Here's how the part is built. I have some questions about the finished solid (model axes, mm). Face numbers are marked on the shaded views. A direction names the side the tool comes from. Round coordinates to 2 decimals unless told otherwise and drop trailing zeros. Write each loop counter-clockwise with the first axis right and the second up, starting at its lowest first coordinate (ties: lowest second). Pieces come first, ordered by that corner, then holes. Notation, with made-up numbers: M 38.5,56.5 L 56.5,56.5 A15 ccw 56.5,83.5 Z; hole C -5.5,58.25 d11. An arc over 180 degrees is marked long. Use a Markdown table: item, result. Add a question column.
```python
from build123d import *

# Parameters (mm, degrees)
F1_DEPTH = 10
F0_R     = 38.1
F0_R_2   = 6.35
F0_R_3   = 5.8823611715
F2_DEPTH = 3
F0_R_4   = 4
F3_DEPTH = 6.35


with BuildPart() as f1:
    # F0 (on Top) → F1 (new body)
    with BuildSketch(Plane.XY):
        with BuildLine():
            Line((25.7629516235, 0), (28.75, 0))
            ThreePointArc((28.75, 0), (28.7346354423, 0.9398010419), (28.6885581914, 1.878597588))
            ThreePointArc((28.6885581914, 1.878597588), (27.1771412956, 2.3608673988), (25.7015098149, 1.7782209055))
            ThreePointArc((25.7015098149, 1.7782209055), (25.7475865895, 0.889641035), (25.7629516235, 0))
        make_face()
        with BuildLine():
            ThreePointArc((28.6885581914, 1.878597588), (28.7346354423, 0.9398010419), (28.75, 0))
            ThreePointArc((28.75, 0), (28.7346354423, -0.9398010419), (28.6885581914, -1.878597588))
            ThreePointArc((28.6885581914, -1.878597588), (29.3734139116, -1.0481230469), (29.6186758117, 0))
            ThreePointArc((29.6186758117, 0), (29.3734139116, 1.0481230469), (28.6885581914, 1.878597588))
        make_face()
        with BuildLine():
            ThreePointArc((28.6885581914, -1.878597588), (28.7346354423, -0.9398010419), (28.75, 0))
            Line((28.75, 0), (25.7629516235, 0))
            ThreePointArc((25.7629516235, 0), (25.7475865895, -0.889641035), (25.7015098149, -1.7782209055))
            ThreePointArc((25.7015098149, -1.7782209055), (27.1771412956, -2.3608673988), (28.6885581914, -1.878597588))
        make_face()
        with BuildLine():
            ThreePointArc((25.7015098149, 1.7782209055), (27.1771412956, 2.3608673988), (28.6885581914, 1.878597588))
            ThreePointArc((28.6885581914, 1.878597588), (20.3293199591, 20.3293199591), (1.878597588, 28.6885581914))
            ThreePointArc((1.878597588, 28.6885581914), (2.2380361997, 28.0122421835), (2.3622, 27.2564758117))
            ThreePointArc((2.3622, 27.2564758117), (2.2113912208, 26.4259713213), (1.7782209055, 25.7015098149))
            ThreePointArc((1.7782209055, 25.7015098149), (18.2171577963, 18.2171577963), (25.7015098149, 1.7782209055))
        make_face()
        with BuildLine():
            ThreePointArc((1.878597588, -28.6885581914), (20.3293199591, -20.3293199591), (28.6885581914, -1.878597588))
            ThreePointArc((28.6885581914, -1.878597588), (27.1771412956, -2.3608673988), (25.7015098149, -1.7782209055))
            ThreePointArc((25.7015098149, -1.7782209055), (18.2171577963, -18.2171577963), (1.7782209055, -25.7015098149))
            ThreePointArc((1.7782209055, -25.7015098149), (2.2113912208, -26.4259713213), (2.3622, -27.2564758117))
            ThreePointArc((2.3622, -27.2564758117), (2.2380361997, -28.0122421835), (1.878597588, -28.6885581914))
        make_face()
        with BuildLine():
            ThreePointArc((25.7015098149, -1.7782209055), (25.7475865895, -0.889641035), (25.7629516235, 0))
            ThreePointArc((25.7629516235, 0), (25.7475865895, 0.889641035), (25.7015098149, 1.7782209055))
            ThreePointArc((25.7015098149, 1.7782209055), (24.8942758117, 0), (25.7015098149, -1.7782209055))
        make_face()
        with BuildLine():
            ThreePointArc((2.3622, 27.2564758117), (2.2380361997, 28.0122421835), (1.878597588, 28.6885581914))
            ThreePointArc((1.878597588, 28.6885581914), (0.9398010419, 28.7346354423), (0, 28.75))
            Line((0, 28.75), (0, 25.7629516235))
            ThreePointArc((0, 25.7629516235), (0.889641035, 25.7475865895), (1.7782209055, 25.7015098149))
            ThreePointArc((1.7782209055, 25.7015098149), (2.2113912208, 26.4259713213), (2.3622, 27.2564758117))
        make_face()
        with BuildLine():
            ThreePointArc((0, 28.75), (0.9398010419, 28.7346354423), (1.878597588, 28.6885581914))
            ThreePointArc((1.878597588, 28.6885581914), (0, 29.6186758117), (-1.878597588, 28.6885581914))
            ThreePointArc((-1.878597588, 28.6885581914), (-0.9398010419, 28.7346354423), (0, 28.75))
        make_face()
        with BuildLine():
            ThreePointArc((-1.878597588, -28.6885581914), (0, -29.6186758117), (1.878597588, -28.6885581914))
            ThreePointArc((1.878597588, -28.6885581914), (0.9398010419, -28.7346354423), (0, -28.75))
            ThreePointArc((0, -28.75), (-0.9398010419, -28.7346354423), (-1.878597588, -28.6885581914))
        make_face()
        with BuildLine():
            ThreePointArc((0, -28.75), (0.9398010419, -28.7346354423), (1.878597588, -28.6885581914))
            ThreePointArc((1.878597588, -28.6885581914), (2.2380361997, -28.0122421835), (2.3622, -27.2564758117))
            ThreePointArc((2.3622, -27.2564758117), (2.2113912208, -26.4259713213), (1.7782209055, -25.7015098149))
            ThreePointArc((1.7782209055, -25.7015098149), (0.889641035, -25.7475865895), (0, -25.7629516235))
            Line((0, -25.7629516235), (0, -28.75))
        make_face()
        with BuildLine():
            Line((0, 25.7629516235), (0, 28.75))
            ThreePointArc((0, 28.75), (-0.9398010419, 28.7346354423), (-1.878597588, 28.6885581914))
            ThreePointArc((-1.878597588, 28.6885581914), (-2.3608673988, 27.1771412956), (-1.7782209055, 25.7015098149))
            ThreePointArc((-1.7782209055, 25.7015098149), (-0.889641035, 25.7475865895), (0, 25.7629516235))
        make_face()
        with BuildLine():
            ThreePointArc((-1.7782209055, 25.7015098149), (-2.3608673988, 27.1771412956), (-1.878597588, 28.6885581914))
            ThreePointArc((-1.878597588, 28.6885581914), (-20.3293199591, 20.3293199591), (-28.6885581914, 1.878597588))
            ThreePointArc((-28.6885581914, 1.878597588), (-27.1771412956, 2.3608673988), (-25.7015098149, 1.7782209055))
            ThreePointArc((-25.7015098149, 1.7782209055), (-18.2171577963, 18.2171577963), (-1.7782209055, 25.7015098149))
        make_face()
        with BuildLine():
            ThreePointArc((-1.7782209055, 25.7015098149), (0, 24.8942758117), (1.7782209055, 25.7015098149))
            ThreePointArc((1.7782209055, 25.7015098149), (0.889641035, 25.7475865895), (0, 25.7629516235))
            ThreePointArc((0, 25.7629516235), (-0.889641035, 25.7475865895), (-1.7782209055, 25.7015098149))
        make_face()
        with BuildLine():
            ThreePointArc((-1.878597588, -28.6885581914), (-0.9398010419, -28.7346354423), (0, -28.75))
            Line((0, -28.75), (0, -25.7629516235))
            ThreePointArc((0, -25.7629516235), (-0.889641035, -25.7475865895), (-1.7782209055, -25.7015098149))
            ThreePointArc((-1.7782209055, -25.7015098149), (-2.3608673988, -27.1771412956), (-1.878597588, -28.6885581914))
        make_face()
        with BuildLine():
            ThreePointArc((-28.6885581914, -1.878597588), (-20.3293199591, -20.3293199591), (-1.878597588, -28.6885581914))
            ThreePointArc((-1.878597588, -28.6885581914), (-2.3608673988, -27.1771412956), (-1.7782209055, -25.7015098149))
            ThreePointArc((-1.7782209055, -25.7015098149), (-18.2171577963, -18.2171577963), (-25.7015098149, -1.7782209055))
            ThreePointArc((-25.7015098149, -1.7782209055), (-27.1771412956, -2.3608673988), (-28.6885581914, -1.878597588))
        make_face()
        with BuildLine():
            ThreePointArc((0, -25.7629516235), (0.889641035, -25.7475865895), (1.7782209055, -25.7015098149))
            ThreePointArc((1.7782209055, -25.7015098149), (0, -24.8942758117), (-1.7782209055, -25.7015098149))
            ThreePointArc((-1.7782209055, -25.7015098149), (-0.889641035, -25.7475865895), (0, -25.7629516235))
        make_face()
        with BuildLine():
            ThreePointArc((-25.7015098149, 1.7782209055), (-27.1771412956, 2.3608673988), (-28.6885581914, 1.878597588))
            ThreePointArc((-28.6885581914, 1.878597588), (-28.7346354423, 0.9398010419), (-28.75, 0))
            Line((-28.75, 0), (-25.7629516235, 0))
            ThreePointArc((-25.7629516235, 0), (-25.7475865895, 0.889641035), (-25.7015098149, 1.7782209055))
        make_face()
        with BuildLine():
            ThreePointArc((-28.75, 0), (-28.7346354423, 0.9398010419), (-28.6885581914, 1.878597588))
            ThreePointArc((-28.6885581914, 1.878597588), (-29.6186758117, 0), (-28.6885581914, -1.878597588))
            ThreePointArc((-28.6885581914, -1.878597588), (-28.7346354423, -0.9398010419), (-28.75, 0))
        make_face()
        with BuildLine():
            ThreePointArc((-28.75, 0), (-28.7346354423, -0.9398010419), (-28.6885581914, -1.878597588))
            ThreePointArc((-28.6885581914, -1.878597588), (-27.1771412956, -2.3608673988), (-25.7015098149, -1.7782209055))
            ThreePointArc((-25.7015098149, -1.7782209055), (-25.7475865895, -0.889641035), (-25.7629516235, 0))
            Line((-25.7629516235, 0), (-28.75, 0))
        make_face()
        with BuildLine():
            ThreePointArc((-24.8942758117, 0), (-25.1055307267, 0.9764343711), (-25.7015098149, 1.7782209055))
            ThreePointArc((-25.7015098149, 1.7782209055), (-25.7475865895, 0.889641035), (-25.7629516235, 0))
            ThreePointArc((-25.7629516235, 0), (-25.7475865895, -0.889641035), (-25.7015098149, -1.7782209055))
            ThreePointArc((-25.7015098149, -1.7782209055), (-25.1055307267, -0.9764343711), (-24.8942758117, 0))
        make_face()
    extrude(amount=-F1_DEPTH)

    # F0 (on Top) → F2 (join)
    with BuildSketch(Plane.XY):
        Circle(F0_R)
        with BuildLine():
            ThreePointArc((1.878597588, 28.6885581914), (20.3293199591, 20.3293199591), (28.6885581914, 1.878597588))
            ThreePointArc((28.6885581914, 1.878597588), (29.3734139116, 1.0481230469), (29.6186758117, 0))
            ThreePointArc((29.6186758117, 0), (29.3734139116, -1.0481230469), (28.6885581914, -1.878597588))
            ThreePointArc((28.6885581914, -1.878597588), (20.3293199591, -20.3293199591), (1.878597588, -28.6885581914))
            ThreePointArc((1.878597588, -28.6885581914), (0, -29.6186758117), (-1.878597588, -28.6885581914))
            ThreePointArc((-1.878597588, -28.6885581914), (-20.3293199591, -20.3293199591), (-28.6885581914, -1.878597588))
            ThreePointArc((-28.6885581914, -1.878597588), (-29.6186758117, 0), (-28.6885581914, 1.878597588))
            ThreePointArc((-28.6885581914, 1.878597588), (-20.3293199591, 20.3293199591), (-1.878597588, 28.6885581914))
            ThreePointArc((-1.878597588, 28.6885581914), (0, 29.6186758117), (1.878597588, 28.6885581914))
        make_face(mode=Mode.SUBTRACT)
        with BuildLine():
            ThreePointArc((25.7015098149, -1.7782209055), (24.8942758117, 0), (25.7015098149, 1.7782209055))
            ThreePointArc((25.7015098149, 1.7782209055), (18.2171577963, 18.2171577963), (1.7782209055, 25.7015098149))
            ThreePointArc((1.7782209055, 25.7015098149), (0, 24.8942758117), (-1.7782209055, 25.7015098149))
            ThreePointArc((-1.7782209055, 25.7015098149), (-18.2171577963, 18.2171577963), (-25.7015098149, 1.7782209055))
            ThreePointArc((-25.7015098149, 1.7782209055), (-25.1055307267, 0.9764343711), (-24.8942758117, 0))
            ThreePointArc((-24.8942758117, 0), (-25.1055307267, -0.9764343711), (-25.7015098149, -1.7782209055))
            ThreePointArc((-25.7015098149, -1.7782209055), (-18.2171577963, -18.2171577963), (-1.7782209055, -25.7015098149))
            ThreePointArc((-1.7782209055, -25.7015098149), (0, -24.8942758117), (1.7782209055, -25.7015098149))
            ThreePointArc((1.7782209055, -25.7015098149), (18.2171577963, -18.2171577963), (25.7015098149, -1.7782209055))
        make_face()
        with Locations((0, -14.8814758117)):
            Circle(F0_R_2, mode=Mode.SUBTRACT)
        with Locations((-14.8917516235, 0)):
            Circle(F0_R_2, mode=Mode.SUBTRACT)
        Circle(F0_R_3, mode=Mode.SUBTRACT)
        with Locations((14.8917516235, 0)):
            Circle(F0_R_2, mode=Mode.SUBTRACT)
        with Locations((0, 14.8814758117)):
            Circle(F0_R_2, mode=Mode.SUBTRACT)
    extrude(amount=-F2_DEPTH)

    # F0 (on Top) → F3 (join)
    with BuildSketch(Plane.XY):
        Circle(F0_R_3)
        Circle(F0_R_4, mode=Mode.SUBTRACT)
    extrude(amount=-F3_DEPTH)


solid = f1.part
```
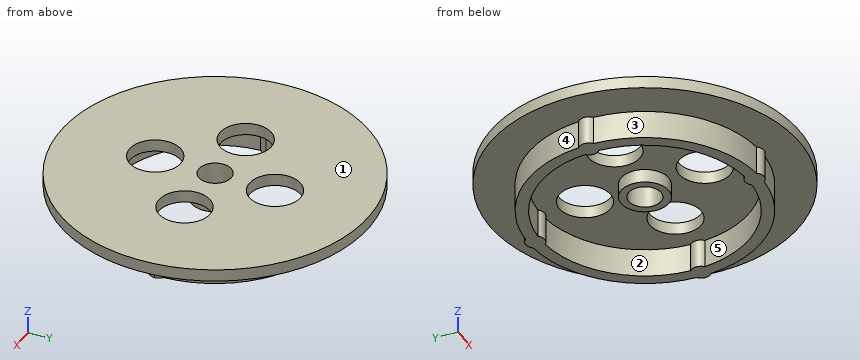
Item 1: On a 3-axis mill with a long thin cutter (end or side, diameter ignored), from which of +Z, -Z, +X, -X, +Y, -Y can I reach the whole of each face in a straight line? I mean the marked faces 1 and 2. Say none if no direction works.
Item 2: Imagine slicing it at B-B on x = 0. List the corners of the cut face in (y, z) for me, plus the area to 3 significant figures.
Item 3: I need wall thicknesses on probe 1 along Y at (x, z) = (0, -1.1); probe 2 along Z at (x, y) = (15, -9); probe 3 along X at (y, z) = (-5, -4.25). Which ranges of each line are inside material? Lowest first, please. Write a range as from..to.
Item 4: Imagine slicing it at D-D on y = -13. List the corners of the cut face in (x, z) for me.
Item 5: If we mould it in two halves opening along Y, with no side actions, what happens to the marked faces 3, 4 and 5? For each: +Y half, -Y half, draft (parallel to the pull), parting line (faces both ways), or undercut.
Item 6: Imagine slicing it at C-C on x = -10.5. List the corners of the cut face in (y, z) for me.
Item 7: For pin 1 Ø6 at (x, y) = (-0.5, 2) entering from -Z; pin 2 Ø5 at (y, z) = (-15, -8) entering from +X; pin 3 Ø2 at (x, y) = (30.5, -23.5) entering from -Z, each with a flat end and sliding along its axis, tell me the tip position at first contact or that it passes through.
Item 8: Imagine slicing it at A-A on z = -8.25. List the corners of the cut face in (x, y) for me.
The answers:
| question | item | result |
|---|---|---|
| 1 | face 1 | +Z, +X, -X, +Y, -Y |
| 1 | face 2 | -Z |
| 2 | outline | M -38.1,-3 L -29.62,-3 L -29.62,-10 L -24.89,-10 L -24.89,-3 L -21.23,-3 L -21.23,0 L -38.1,0 Z; M -8.53,-3 L -5.88,-3 L -5.88,-6.35 L -4,-6.35 L -4,0 L -8.53,0 Z; M 4,-6.35 L 5.88,-6.35 L 5.88,-3 L 8.53,-3 L 8.53,0 L 4,0 Z; M 21.23,-3 L 24.89,-3 L 24.89,-10 L 29.62,-10 L 29.62,-3 L 38.1,-3 L 38.1,0 L 21.23,0 Z |
| 2 | area | 207 mm² |
| 3 | probe 1 | -38.1..-21.23, -8.53..-4, 4..8.53, 21.23..38.1 |
| 3 | probe 2 | -3..0 |
| 3 | probe 3 | -28.31..-25.27, -3.1..3.1, 25.27..28.31 |
| 4 | outline | M -35.81,-3 L -25.64,-3 L -25.64,-10 L -22.24,-10 L -22.24,-3 L -6.06,-3 L -6.06,0 L -35.81,0 Z; M 6.06,-3 L 22.24,-3 L 22.24,-10 L 25.64,-10 L 25.64,-3 L 35.81,-3 L 35.81,0 L 6.06,0 Z |
| 5 | face 3 | -Y half |
| 5 | face 4 | +Y half |
| 5 | face 5 | undercut |
| 6 | outline | M -36.62,-3 L -26.76,-3 L -26.76,-10 L -23.53,-10 L -23.53,-3 L -4.59,-3 L -4.59,0 L -36.62,0 Z; M 4.59,-3 L 23.53,-3 L 23.53,-10 L 26.76,-10 L 26.76,-3 L 36.62,-3 L 36.62,0 L 4.59,0 Z |
| 7 | pin 1 | z = -6.35 |
| 7 | pin 2 | x = 25.89 |
| 7 | pin 3 | z = -3 |
| 8 | outline | M -28.69,-1.88 A28.75 ccw -1.88,-28.69 A2.36 ccw 1.88,-28.69 A28.75 ccw 28.69,-1.88 A2.36 ccw 28.69,1.88 A28.75 ccw 1.88,28.69 A2.36 ccw -1.88,28.69 A28.75 ccw -28.69,1.88 A2.36 ccw Z; hole M -25.7,-1.78 A25.76 ccw -1.78,-25.7 A2.36 cw 1.78,-25.7 A25.76 ccw 25.7,-1.78 A2.36 cw 25.7,1.78 A25.76 ccw 1.78,25.7 A2.36 cw -1.78,25.7 A25.76 ccw -25.7,1.78 A2.36 cw Z |
